Job drawing, mm, ordinate dimensions from the low corner. One solid piece. A direction names the side the tool comes from. Give positions to 0.01 mm unless a question says otherwise; leave off trailing zeros. Loops run counter-clockwise (first coordinate to the right, second up) from the corner with the lowest first, then second, coordinate; pieces in that order, holes last. Notation, with made-up numbers: M 35,31 L 81,31 A23 ccw 81,56 Z; hole C 37.5,-1 d7. An arc over 180 degrees is marked long. Put each result on its own line as item: value.
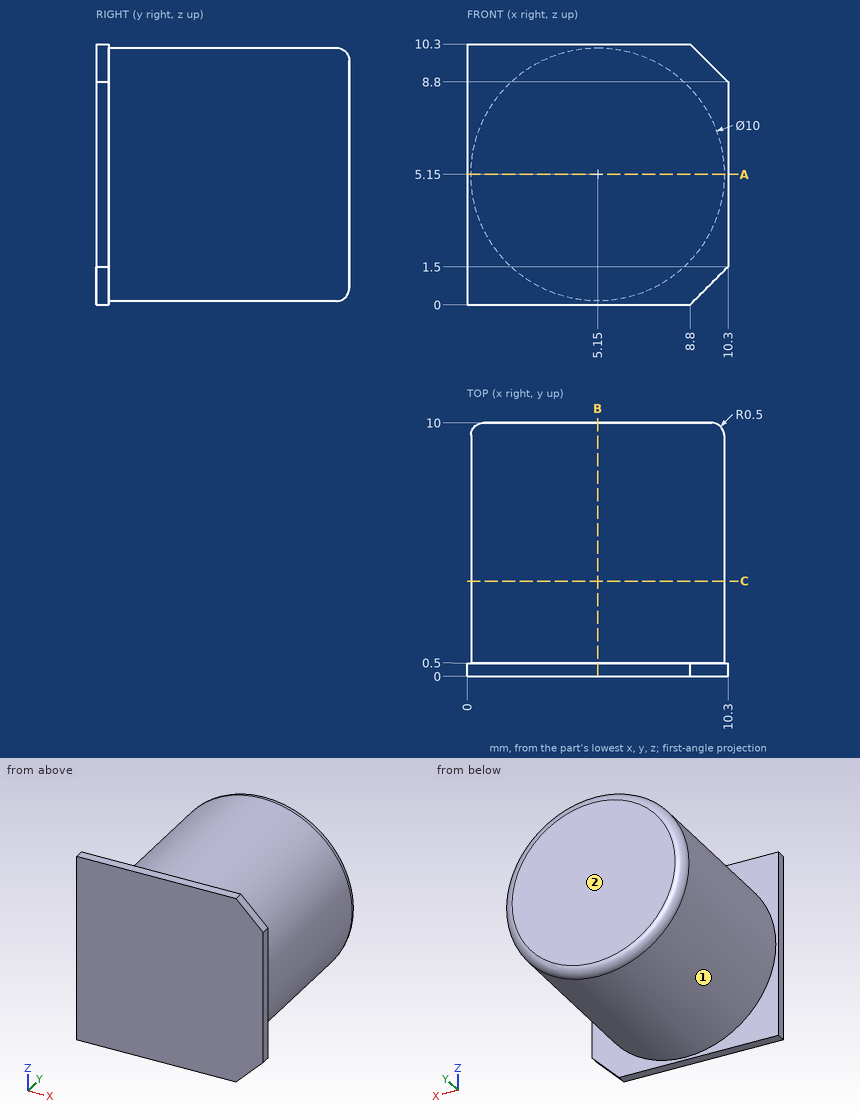
Q1. Slice it at B-B (x = 5.15). List the corners of the cut face in (y, z).
Here are the results:
outline: M 0,0 L 0.5,0 L 0.5,0.15 L 9.5,0.15 A0.5 ccw 10,0.65 L 10,9.65 A0.5 ccw 9.5,10.15 L 0.5,10.15 L 0.5,10.3 L 0,10.3 Z
Q2. Drop flat-ended pins along their axis: pin 1 Ø6 at (y, z) = (4, 3.5) entering from +X; pin 2 Ø6 at (y, z) = (6.5, 7.5) entering from -X. Give the stop position or say it passes through.
Here are the results:
pin 1: x = 10.15
pin 2: x = 0.15
Q3. Tool access for the marked faces 1 and 2: list every direction of +Z, -Z, +X, -X, +Y, -Y with a clear straight run to the whole face (end or side of a thin tool).
Here are the results:
face 1: +Y
face 2: +Z, -Z, +X, -X, +Y
Q4. Slice it at A-A (z = 5.15). List the corners of the cut face in (x, y).
Here are the results:
outline: M 0,0 L 10.3,0 L 10.3,0.5 L 10.15,0.5 L 10.15,9.5 A0.5 ccw 9.65,10 L 0.65,10 A0.5 ccw 0.15,9.5 L 0.15,0.5 L 0,0.5 Z
Q5. Slice it at C-C (y = 3.75). List the corners of the cut face in (x, z).
Here are the results:
outline: C 5.15,5.15 d10
Q6. Probe line 1 (Y direction, x = 6.25, z = 0.75); line 2 (X direction, y = 8.5, z = 5); line 3 (Y direction, x = 9.25, z = 2). List the from-to ranges inside material, lowest first. Write a range as from..to.
Here are the results:
line 1: 0..10
line 2: 0.15..10.15
line 3: 0..0.5
